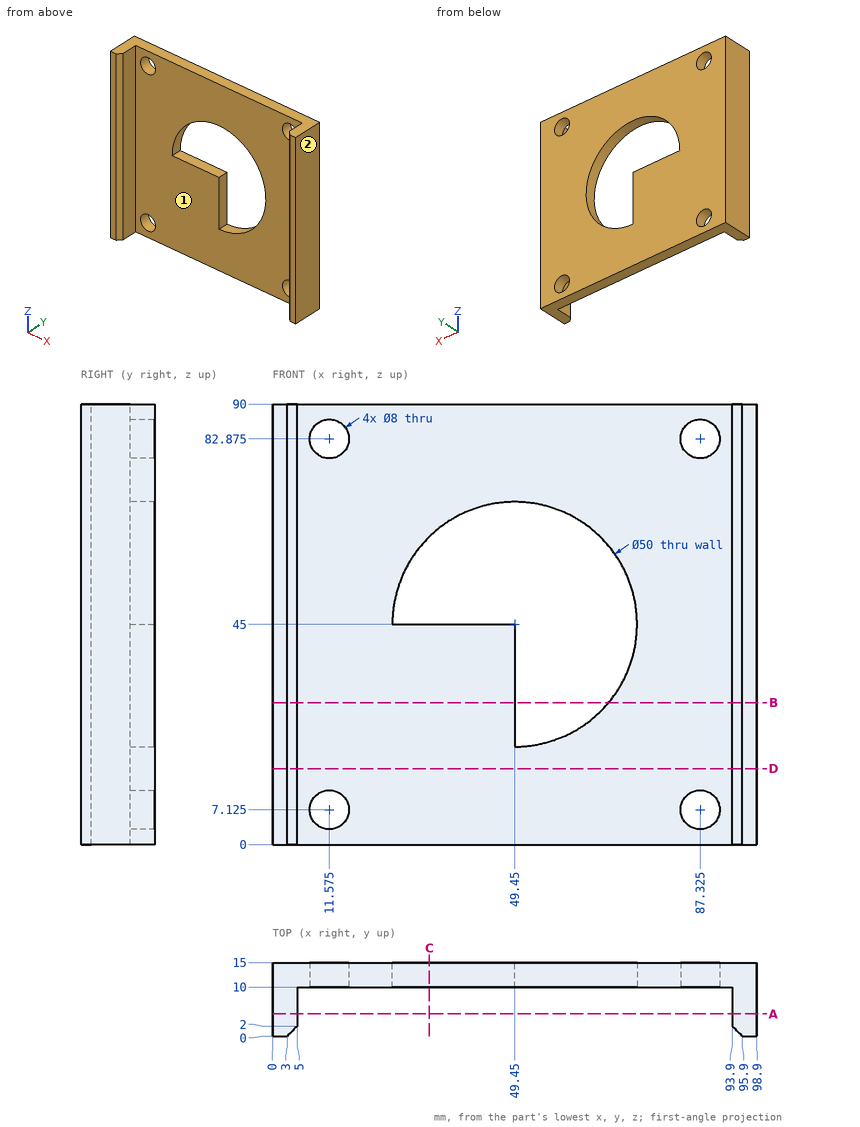
Input: dimensioned drawing with shaded views. Units: mm. Origin: part minimum x, y, z. A direction names the side the tool comes from. Give positions to 0.01 mm unless a question says otherwise; leave off trailing zeros. Write each loop counter-clockwise with the first axis right and the second up, starting at its lowest first coordinate (ties: lowest second). Pieces come first, ordered by that corner, then holes.
Q1. Section D-D, the plane z = 15.5. Output: boundary loops of the cut face in (x, y), plus the area to 4 significant figures.
Q2. Section C-C, the plane x = 32. Output: boundary loops of the cut face in (y, z), plus the area to 3 significant figures.
Q3. Section B-B, the plane z = 29. Output: boundary loops of the cut face in (x, y), plus the area to 3 significant figures.
Q4. Section A-A, the plane y = 4.5. Output: boundary loops of the cut face in (x, z).
Q5. Set-up query: the marked faces 1 and 2. Return all of +Z, -Z, +X, -X, +Y, -Y with unobstructed straight access to the full face (end or side cutting, diameter ignored); none if empty.
Q6. First-contact query: P1, Ø5, axis at x = 11.575, z = 82.875, coming from the -Y side; P2, Ø1, axis at x = 15, z = 46, coming from the -Y side. Flat tips, straight axial feed; report the tip coordinate or a pass-through.
Q7. Material intervals for probe 1 along X at (y, z) = (7.75, 83); probe 2 along X at (y, z) = (11.5, 8); probe 3 along Y at (x, z) = (14, 57), sorted ascending.
Filled in:
1. outline: (0, 0) - (3, 0) - (5, 2) - (5, 10) - (93.9, 10) - (93.9, 2) - (95.9, 0) - (98.9, 0) - (98.9, 15) - (0, 15) - close
1. area: 590.5 mm2
2. outline: (10, 0) - (15, 0) - (15, 45) - (10, 45) - close; (10, 62.9) - (15, 62.9) - (15, 90) - (10, 90) - close
2. area: 360 mm2
3. outline: (0, 0) - (3, 0) - (5, 2) - (5, 10) - (49.45, 10) - (49.45, 15) - (0, 15) - close; (68.66, 10) - (93.9, 10) - (93.9, 2) - (95.9, 0) - (98.9, 0) - (98.9, 15) - (68.66, 15) - close
3. area: 494 mm2
4. outline: (0, 0) - (5, 0) - (5, 90) - (0, 90) - close; (93.9, 0) - (98.9, 0) - (98.9, 90) - (93.9, 90) - close
5. face 1: +Z, -Z, -Y
5. face 2: +Z, -Z, +X, +Y, -Y
6. P1: passes through
6. P2: stops at y = 10
7. probe 1: x = 0 to 5, 93.9 to 98.9
7. probe 2: x = 0 to 7.67, 15.48 to 83.42, 91.23 to 98.9
7. probe 3: y = 10 to 15
